from build123d import *

# Parameters (mm, degrees)
SKETCH15_R          = 3.3
SKETCH15_R_2        = 2.5
SKETCH15_R_3        = 52.3875
SKETCH15_R_4        = 4.5
SKETCH15_R_5        = 27.4955
BOSS_EXTRUDE1_DEPTH = 7.62
PROFILE_DEPTH       = 804.110776731
PROF_FILLET_R       = 12.7
CUT_EXTRUDE2_DEPTH  = 804.110776731
FILLET2_R           = 6.35
CUT_EXTRUDE4_DEPTH  = 804.110776731
FILLET5_R           = 6.35
CUT_EXTRUDE8_DEPTH  = 804.110776731
FILLET6_R           = 12.7


with BuildPart() as part:
    # Sketch15 → Boss-Extrude1 (new body)
    with BuildSketch(Plane(origin=(0, 0, 0), x_dir=(-1, 0, 0), z_dir=(0, 0, 1))):
        with BuildLine():
            ThreePointArc((-776.492771968, 151.978917225), (-781.907485254, 150.230614898), (-784.225, 145.034))
            Line((-784.225, 145.034), (-784.225, 0))
            ThreePointArc((-784.225, 0), (-782.179140867, -4.939140867), (-777.24, -6.985))
            Line((-777.24, -6.985), (-548.64, -6.985))
            ThreePointArc((-548.64, -6.985), (-545.651186694, -6.313257481), (-543.237237519, -4.427231931))
            Line((-543.237237519, -4.427231931), (-459.418508663, 97.860764379))
            ThreePointArc((-459.418508663, 97.860764379), (-449.426249212, 133.212914363), (-468.520845097, 164.597881552))
            ThreePointArc((-468.520845097, 164.597881552), (-470.201009111, 165.051242365), (-471.778645707, 164.316701751))
            Line((-471.778645707, 164.316701751), (-477.043529325, 159.051818133))
            ThreePointArc((-477.043529325, 159.051818133), (-484.127165713, 157.642795249), (-488.139723403, 163.648012211))
            Line((-488.139723403, 163.648012211), (-488.139723403, 170.220745001))
            ThreePointArc((-488.139723403, 170.220745001), (-488.796888696, 171.925600851), (-490.428332433, 172.748273949))
            ThreePointArc((-490.428332433, 172.748273949), (-494.978508993, 172.974), (-499.528685552, 172.748273949))
            ThreePointArc((-499.528685552, 172.748273949), (-501.160129289, 171.925600851), (-501.817294582, 170.220745001))
            Line((-501.817294582, 170.220745001), (-501.817294582, 163.648012211))
            ThreePointArc((-501.817294582, 163.648012211), (-508.317294582, 157.148012211), (-514.817294582, 163.648012211))
            Line((-514.817294582, 163.648012211), (-514.817294582, 164.225022653))
            ThreePointArc((-514.817294582, 164.225022653), (-516.106794745, 166.435870942), (-518.665995494, 166.401924563))
            Line((-518.665995494, 166.401924563), (-660.126842441, 139.458698233))
            Line((-660.126842441, 139.458698233), (-776.492771968, 151.978917225))
        make_face()
        with Locations((-777.24, 0)):
            Circle(SKETCH15_R, mode=Mode.SUBTRACT)
        with Locations((-709.220726776, 39.660663218)):
            Circle(SKETCH15_R_2, mode=Mode.SUBTRACT)
        with Locations((-666.75, 20.751477371)):
            Circle(SKETCH15_R_2, mode=Mode.SUBTRACT)
        with Locations((-624.279273224, 39.660663218)):
            Circle(SKETCH15_R_2, mode=Mode.SUBTRACT)
        with Locations((-666.75, 77.901477371)):
            Circle(SKETCH15_R_3, mode=Mode.SUBTRACT)
        with Locations((-548.64, 0)):
            Circle(SKETCH15_R, mode=Mode.SUBTRACT)
        with Locations((-723.58692632, 83.875279047)):
            Circle(SKETCH15_R_2, mode=Mode.SUBTRACT)
        with Locations((-709.220726776, 116.142291524)):
            Circle(SKETCH15_R_2, mode=Mode.SUBTRACT)
        with Locations((-628.509185847, 120.372204147)):
            Circle(SKETCH15_R_2, mode=Mode.SUBTRACT)
        with Locations((-777.24, 145.034)):
            Circle(SKETCH15_R, mode=Mode.SUBTRACT)
        with Locations((-666.75, 135.051477371)):
            Circle(SKETCH15_R_2, mode=Mode.SUBTRACT)
        with Locations((-609.91307368, 83.875279047)):
            Circle(SKETCH15_R_2, mode=Mode.SUBTRACT)
        with Locations((-508.317294582, 90.351987789)):
            Circle(SKETCH15_R_4, mode=Mode.SUBTRACT)
        with Locations((-481.639723403, 90.351987789)):
            Circle(SKETCH15_R_4, mode=Mode.SUBTRACT)
        with Locations((-528.75349974, 107.5)):
            Circle(SKETCH15_R_4, mode=Mode.SUBTRACT)
        with Locations((-494.978508993, 127)):
            Circle(SKETCH15_R_5, mode=Mode.SUBTRACT)
        with Locations((-461.203518245, 107.5)):
            Circle(SKETCH15_R_4, mode=Mode.SUBTRACT)
        with Locations((-533.38601136, 133.772278929)):
            Circle(SKETCH15_R_4, mode=Mode.SUBTRACT)
        with Locations((-456.571006625, 133.772278929)):
            Circle(SKETCH15_R_4, mode=Mode.SUBTRACT)
        with Locations((-520.04722577, 156.875733282)):
            Circle(SKETCH15_R_4, mode=Mode.SUBTRACT)
        with Locations((-494.978508993, 166)):
            Circle(SKETCH15_R_4, mode=Mode.SUBTRACT)
        with Locations((-469.909792215, 156.875733282)):
            Circle(SKETCH15_R_4, mode=Mode.SUBTRACT)
    extrude(amount=BOSS_EXTRUDE1_DEPTH)

    # Sketch18 → Profile (cut, through all)
    with BuildSketch(Plane.XY.offset(7.62)):
        with BuildLine():
            Line((656.843849148, -10.682497906), (776.22161066, 6.910362375))
            ThreePointArc((776.22161066, 6.910362375), (776.729439616, 6.966315604), (777.24, 6.985))
            Line((777.24, 6.985), (548.64, 6.985))
            ThreePointArc((548.64, 6.985), (549.207578223, 6.961902036), (549.771402717, 6.892760905))
            Line((549.771402717, 6.892760905), (656.843849148, -10.682497906))
        make_face()
        with BuildLine():
            Line((735.827075043, -69.956273799), (783.061059407, -141.173236814))
            ThreePointArc((783.061059407, -141.173236814), (783.927687379, -143.01779998), (784.225, -145.034))
            Line((784.225, -145.034), (784.225, 0))
            ThreePointArc((784.225, 0), (783.891483704, -2.132601588), (782.922783957, -4.061550382))
            Line((782.922783957, -4.061550382), (735.827075043, -69.956273799))
        make_face()
    extrude(amount=-PROFILE_DEPTH, mode=Mode.SUBTRACT)

    # Prof Fillet
    prof_fillet_edges = [part.edges().sort_by_distance(p)[0] for p in [
        (656.843849148, -10.682497906, 3.81),
        (660.126842441, -139.458698233, 3.81),
    ]]
    fillet(prof_fillet_edges, radius=PROF_FILLET_R)

    # Sketch19 → Cut-Extrude2 (cut, through all)
    with BuildSketch(Plane.XY.offset(7.62)):
        with BuildLine():
            Line((733.394654999, -58.070730629), (773.084551456, -2.537969581))
            Line((773.084551456, -2.537969581), (694.45302227, -14.12600314))
            ThreePointArc((694.45302227, -14.12600314), (718.789944466, -31.786265822), (733.394654999, -58.070730629))
        make_face()
        with BuildLine():
            Line((735.555674658, -87.928824534), (772.681244896, -143.90484261))
            Line((772.681244896, -143.90484261), (704.133403657, -136.529539656))
            ThreePointArc((704.133403657, -136.529539656), (725.141244771, -115.65371029), (735.555674658, -87.928824534))
        make_face()
    extrude(amount=-CUT_EXTRUDE2_DEPTH, mode=Mode.SUBTRACT)

    # Fillet2
    fillet2_edges = [part.edges().sort_by_distance(p)[0] for p in [
        (735.555674658, -87.928824534, 3.81),
        (772.681244896, -143.90484261, 3.81),
        (704.133403657, -136.529539656, 3.81),
        (773.084551456, -2.537969581, 3.81),
        (733.394654999, -58.070730629, 3.81),
        (694.45302227, -14.12600314, 3.81),
    ]]
    fillet(fillet2_edges, radius=FILLET2_R)

    # Sketch22 → Cut-Extrude4 (cut, through all)
    with BuildSketch(Plane.XY.offset(7.62)):
        with BuildLine():
            Line((632.611679529, -14.426912925), (566.137854436, -3.515658731))
            Line((566.137854436, -3.515658731), (544.206709687, -14.426912925))
            Line((544.206709687, -14.426912925), (505.79558687, -61.301839836))
            Line((505.79558687, -61.301839836), (596.214449629, -63.096701449))
            ThreePointArc((596.214449629, -63.096701449), (609.03222208, -34.737796246), (632.611679529, -14.426912925))
        make_face()
        with BuildLine():
            Line((630.634467741, -137.318957004), (546.092983647, -153.421082711))
            Line((546.092983647, -153.421082711), (598.051124974, -88.636146739))
            ThreePointArc((598.051124974, -88.636146739), (608.965754764, -116.576398946), (630.634467741, -137.318957004))
        make_face()
        with BuildLine():
            Line((502.723422183, -71.402857307), (600.547071221, -73.344707791))
            Line((600.547071221, -73.344707791), (550.408802524, -135.86050309))
            ThreePointArc((550.408802524, -135.86050309), (540.105814597, -93.615089563), (502.723422183, -71.402857307))
        make_face()
    extrude(amount=-CUT_EXTRUDE4_DEPTH, mode=Mode.SUBTRACT)

    # Fillet5
    fillet5_edges = [part.edges().sort_by_distance(p)[0] for p in [
        (566.137854436, -3.515658731, 3.81),
        (544.206709687, -14.426912925, 3.81),
        (505.79558687, -61.301839836, 3.81),
        (596.214449629, -63.096701449, 3.81),
        (632.611679529, -14.426912925, 3.81),
        (502.723422183, -71.402857307, 3.81),
        (600.547071221, -73.344707791, 3.81),
        (550.408802524, -135.86050309, 3.81),
        (630.634467741, -137.318957004, 3.81),
        (546.092983647, -153.421082711, 3.81),
        (598.051124974, -88.636146739, 3.81),
    ]]
    fillet(fillet5_edges, radius=FILLET5_R)

    # Sketch26 → Cut-Extrude8 (cut, through all)
    with BuildSketch(Plane.XY.offset(7.62)):
        with BuildLine():
            Line((735.555674658, -87.928824534), (772.681244896, -143.90484261))
            Line((772.681244896, -143.90484261), (704.133403657, -136.529539656))
            ThreePointArc((704.133403657, -136.529539656), (698.023230979, -140.004243657), (691.593468887, -142.844303071))
            Line((691.593468887, -142.844303071), (776.492771968, -151.978917225))
            ThreePointArc((776.492771968, -151.978917225), (783.208804193, -148.662167789), (783.061059407, -141.173236814))
            Line((783.061059407, -141.173236814), (735.827075043, -69.956273799))
            ThreePointArc((735.827075043, -69.956273799), (736.168550391, -73.922354613), (736.2825, -77.901477371))
            ThreePointArc((736.2825, -77.901477371), (736.100555619, -82.928304557), (735.555674658, -87.928824534))
        make_face()
        with BuildLine():
            ThreePointArc((704.133403657, -136.529539656), (725.141244771, -115.65371029), (735.555674658, -87.928824534))
            Line((735.555674658, -87.928824534), (772.681244896, -143.90484261))
            Line((772.681244896, -143.90484261), (704.133403657, -136.529539656))
        make_face()
        with BuildLine():
            ThreePointArc((704.133403657, -136.529539656), (725.141244771, -115.65371029), (735.555674658, -87.928824534))
            ThreePointArc((735.555674658, -87.928824534), (736.100555619, -82.928304557), (736.2825, -77.901477371))
            ThreePointArc((736.2825, -77.901477371), (736.168550391, -73.922354613), (735.827075043, -69.956273799))
            add(Edge.make_bspline(
                [(662.00549252, -139.660828792), (729.199735591, -143.098901444), (735.827075043, -69.956273799)],
                knots=[0, 0, 0, 1, 1, 1], degree=2))
            Line((662.00549252, -139.660828792), (691.593468887, -142.844303071))
            ThreePointArc((691.593468887, -142.844303071), (698.023230979, -140.004243657), (704.133403657, -136.529539656))
        make_face()
    extrude(amount=-CUT_EXTRUDE8_DEPTH, mode=Mode.SUBTRACT)

    # Fillet6
    fillet6_edges = [part.edges().sort_by_distance(p)[0] for p in [
        (735.827075043, -69.956273799, 3.81),
    ]]
    fillet(fillet6_edges, radius=FILLET6_R)


solid = part.part
Read the model definition and answer for the solid it produces. Units are mm, in the model's axes. A direction names the side the tool comes from. Give positions to 0.01 mm unless a question says otherwise; leave off trailing zeros. Write each loop counter-clockwise with the first axis right and the second up, starting at its lowest first coordinate (ties: lowest second). Pieces come first, ordered by that corner, then holes. Notation, with made-up numbers: (40, -28.5) - (73, -28.5) arc R18 cw to (73, -0.5) - close; hole circle Ø7 at (-3.5, 24). An arc over 180 degrees is marked (long way). Return JSON: item names as keys, results as strings.
Q1. A cutting plane is placed at B-B, the plane x = 649.5. Determine the outline of the cut face in (y, z), and give its area (3 significant figures).
Reply:
{"outline": "(-141.48, 0) - (-127.37, 0) - (-127.37, 7.62) - (-141.48, 7.62) - close; (-28.44, 0) - (-9.48, 0) - (-9.48, 7.62) - (-28.44, 7.62) - close", "area": "252 mm²"}
Q2. Consider line 1 along Y through (x, z) = (560, 2.75); line 2 along X through (y, z) = (-17.5, 2.75); line 3 along X through (y, z) = (-14.5, 1). Determine where each line is inside the solid, lowest interval first. Write a range as [from, to].
Reply:
{"line 1": "[-158.53, -150.05], [-136.08, -123.24], [-72.54, -62.38], [-6.57, 5.21]", "line 2": "[525.27, 541.69], [622.3, 706.73], [762.39, 773.32]", "line 3": "[527.73, 544.35], [621.19, 707.65], [764.53, 775.46]"}
Q3. A cutting plane is placed at C-C, the plane x = 482.5. Determine the outline of the cut face in (y, z).
Reply:
{"outline": "(-157.21, 0) - (-151.5, 0) - (-151.5, 7.62) - (-157.21, 7.62) - close; (-102.5, 0) - (-94.77, 0) - (-94.77, 7.62) - (-102.5, 7.62) - close; (-85.93, 0) - (-69.69, 0) - (-69.69, 7.62) - (-85.93, 7.62) - close"}
Q4. Given P1, Ø1, axis at y = -16.5, z = 1, coming from the +X side; P2, Ø1, axis at y = -104, z = 4.5, coming from the +X side; P3, Ø1.5, axis at x = 636.5, z = 5.5, coming from the -Y side, each flat-ended and moving along its own axis, determine where each tip first touches the part or whether it passes through.
Reply:
{"P1": "x = 774.39", "P2": "x = 727.99", "P3": "y = -144.1"}
Q5. For faces 1 (the face through (587.491, -153.293, 3.757)), 2 (the face through (488.14, -167, 4)), 3 (the face through (554.997, -9.059, 3.863)), determine the directions among +Z, -Z, +X, -X, +Y, -Y from which every point of the face is accessible in a straight line to the end or side of a thin tool.
Reply:
{"face 1": "+Z, -Z, +X, -Y", "face 2": "+Z, -Z, -Y", "face 3": "+Z, -Z"}
Q6. A cutting plane is placed at A-A, the plane y = -146.5. Determine the outline of the cut face in (x, z).
Reply:
{"outline": "(453.34, 0) - (475.59, 0) - (475.59, 7.62) - (453.34, 7.62) - close; (514.36, 0) - (556, 0) - (556, 7.62) - (514.36, 7.62) - close; (582.43, 0) - (623.16, 0) - (623.16, 7.62) - (582.43, 7.62) - close"}
Q7. For a pull along X with two mould halves and no side action, classify faces 4 (the face through (774.09, -0.99, 3.76)), 5 (the face through (556.3, -147.1, 3.8)), 6 (the face through (494.915, -172.974, 3.757)), 7 (the face through (605, -70, 0)) as released by +X, released by -X, zero draft, split by the parting line, or undercut.
Reply:
{"face 4": "undercut", "face 5": "undercut", "face 6": "split by the parting line", "face 7": "zero draft"}
Q8. A cutting plane is placed at D-D, the plane z = 4.25. Count the separate pieces of the cut face and the enclosed holes in it, and give its area (3 significant figures).
Reply:
{"separate pieces": "1", "enclosed holes": "25", "area": "17,200 mm²"}
